Geometry: final body of the model. Coordinates: model frame, mm. A direction names the side the tool comes from. Coordinates: 2 decimals unless noted, no trailing zeros. Write each loop counter-clockwise with the first axis right and the second up, starting at its lowest first coordinate (ties: lowest second). Pieces come first, ordered by that corner, then holes. Notation, with made-up numbers: (8, 23.25) - (30, 23.25) arc R20 ccw to (30, 54.25) - close; hole circle Ø4 at (-13.5, 35). An arc over 180 degrees is marked (long way). Answer as a JSON object with one key per item and string values. Group by question number.
Item 1: Set-up query: faces 1 (the flat face through (7, 12.5, 0)), 2 (the flat face through (1, -35, 4)), 3 (the flat face through (7, 15, -29)). Return all of +Z, -Z, +X, -X, +Y, -Y with unobstructed straight access to the full face (end or side cutting, diameter ignored); none if empty.
Item 2: Section A-A on y = -25. Return loops of the section in (x, z).
Item 3: First-contact query: pin 1 Ø1.5 at (x, z) = (-5.5, -24) entering from -Y; pin 2 Ø10 at (x, z) = (1.5, -12.5) entering from -Y; pin 3 Ø6 at (x, z) = (0, 0) entering from +Y. Flat tips, straight axial feed; report the tip coordinate or a pass-through.
Item 4: Mould query, pull axis Z, two halves, no side actions, for faces 4 (the flat face through (-9.5, 1, 16.7)), 5 (the flat face through (0, -19, 30.5)), 6 (the flat face through (-7, 6, 4.5)). Classes: pulls with the +Z half, pulls with the -Z half, needs draft (parallel to the pull), parting line crosses it, or undercut.
Item 5: Section B-B on y = -39. Return loops of the section in (x, z), and give its area (3 significant figures).
Item 6: Line query: line 1 along X through (y, z) = (7, -6.5); line 2 along Y through (x, z) = (0.5, 17); line 3 along Z through (x, y) = (0, -40.25). Output: solid intervals per line, ascending. Write a range as from..to.
Item 7: Section C-C on z = 12.5. Return loops of the section in (x, y), and give its area (4 significant figures).
Autodesk Inventor part; units mm, degrees
ref_plane "YZ Plane" through (0, 0, 0) normal (1, 0, 0) x (0, 1, 0)
ref_plane "XZ Plane" through (0, 0, 0) normal (0, 1, 0) x (-1, 0, 0)
ref_plane "XY Plane" through (0, 0, 0) normal (0, 0, 1) x (1, 0, 0)
sketch "Sketch1" plane through (0, 0, 0) normal (0, 1, 0) x (-1, 0, 0)
  line L0 (6, 30.5) -> (-6, 30.5)
  line L1 (-6, 30.5) -> (-6, -30.5)
  line L2 (-6, -30.5) -> (6, -30.5)
  line L3 (6, -30.5) -> (6, 30.5)
  line L4 (8.5, 30.5) -> (-8.5, 30.5)
  line L5 (-8.5, 30.5) -> (-8.5, -30.5)
  line L6 (-8.5, -30.5) -> (8.5, -30.5)
  line L7 (8.5, -30.5) -> (8.5, 30.5)
  point P0 (0, 0)
  point P1 (-6, 30.5)
  dimension "d0" = 61
  dimension "d1" = 30.5
  dimension "d2" = 0
  dimension "d3" = 0
  dimension "d4" = 2.5
  dimension "d5" = 2.5
  dimension "d6" = 12
  dimension "d7" = 6
extrude "Extrusion1" add sketch "Sketch1" along normal blind 15.5 contours L4 L7 L6 L3 | L1 L6 L5 L4
sketch "Sketch2" plane through (0, 0, 0) normal (0, 1, 0) x (-1, 0, 0)
  line L0 (-11.5, 28) -> (11.5, 28)
  line L1 (11.5, 28) -> (11.5, -28)
  line L2 (11.5, -28) -> (-11.5, -28)
  line L3 (-11.5, -28) -> (-11.5, 28)
  line L4 (-8.5, 30.5) -> (-8.5, -30.5)
  line L5 (8.5, -30.5) -> (8.5, 30.5)
  point P0 (0, 0)
  dimension "d10" = 56
  dimension "d11" = 28
  dimension "d12" = 3
  dimension "d13" = 3
extrude "Extrusion2" add sketch "Sketch2" against normal blind 2.5
sketch "Sketch3" plane through (0, -2.5, 0) normal (0, -1, 0) x (1, 0, 0)
  line L0 (11.5, -30.5) -> (-11.5, -30.5)
  line L1 (-11.5, -30.5) -> (-11.5, 30.5)
  line L2 (-11.5, 30.5) -> (11.5, 30.5)
  line L3 (11.5, 30.5) -> (11.5, -30.5)
  line L4 (11.5, -28) -> (11.5, 28)
  line L5 (-11.5, 28) -> (-11.5, -28)
  line L6 (-11.5, -28) -> (11.5, -28)
  line L7 (11.5, 28) -> (-11.5, 28)
  point P0 (0, 0)
  point P1 (11.5, -28)
  point P2 (-11.5, -28)
  point P3 (-11.5, 28)
  point P4 (11.5, 28)
  dimension "d16" = 0
  dimension "d17" = 0
  dimension "d18" = 2.5
  dimension "d19" = 2.5
extrude "Extrusion3" add sketch "Sketch3" along normal blind 35 and the other way blind 2.5 contours L0 L1 L6 L3 | L7 L1 L2 L3
sketch "Sketch4" plane through (0, -37.5, 0) normal (0, -1, 0) x (1, 0, 0)
  line L0 (11.5, 30.5) -> (11.5, -30.5)
  line L1 (-11.5, -30.5) -> (-11.5, 30.5)
  line L2 (11.5, -30.5) -> (-11.5, -30.5)
  line L3 (-11.5, -30.5) -> (-11.5, 30.5)
  line L4 (-11.5, 30.5) -> (11.5, 30.5)
  line L5 (11.5, 30.5) -> (11.5, -30.5)
  point P0 (0, 0)
  point P1 (-11.5, -30.5)
extrude "Extrusion4" add sketch "Sketch4" along normal blind 2.5
sketch "Sketch5" plane through (0, -40, 0) normal (0, -1, 0) x (1, 0, 0)
  circle A0 centre (0, 0) radius 6
  dimension "d26" = 12
extrude "Extrusion5" add sketch "Sketch5" along normal blind 3 and the other way blind 6
sketch "Sketch6" plane through (0, -43, 0) normal (0, -1, 0) x (1, 0, 0)
  circle A0 centre (0, 0) radius 3.75
  circle A1 centre (0, 0) radius 5
  dimension "d31" = 7.5
  dimension "d32" = 10
extrude "Extrusion6" cut sketch "Sketch6" against normal blind 8
sketch "Sketch7" plane through (0, 0, 0) normal (0, 1, 0) x (1, 0, 0)
  line L0 (-11.5, -4.5) -> (12.0053, -4.5)
  line L1 (12.0053, -4.5) -> (12.0053, 4.5)
  line L2 (12.0053, 4.5) -> (-11.5, 4.5)
  line L3 (-11.5, 4.5) -> (-11.5, -4.5)
  line L4 (-11.5, 28) -> (-11.5, -28)
  point P0 (0, 0)
  point P1 (-12, 31)
  point P2 (-12, -31)
  dimension "d35" = 0
  dimension "d36" = 9
  dimension "d37" = 4.5
extrude "Extrusion7" cut sketch "Sketch7" along normal blind 12.5
chamfer "Chamfer1" distance 2 angle 45 12 edges at (-7.25, 12.5, 4.5) (-7.25, 0, 4.5) (7.25, 0, 4.5) (7.25, 12.5, -4.5) (7.25, 12.5, 4.5) (-7.25, 12.5, -4.5) (7.25, 0, -4.5) (-7.25, 0, -4.5) (8.5, 0, 17.5) (8.5, 0, -17.5) (-8.5, 0, -17.5) (-8.5, 0, 17.5)
chamfer "Chamfer2" distance 2 angle 45 4 edges at (-7.25, 15.5, 30.5) (7.25, 15.5, 30.5) (-7.25, 15.5, -30.5) (7.25, 15.5, -30.5)
fillet "Fillet1" radius 3 2 edges at (-6, -40, 0) (-6, -37.5, 0)
sketch "Sketch10" plane through (11.5, 0, 30.5) normal (1, 0, 0) x (0, 0, -1)
  line L0 (0, 0) -> (0, -40)
  line L1 (2.5, -37.5) -> (2.5, -2.5)
  line L2 (0, -40) -> (2.5, -37.5)
  line L3 (58.5, -2.5) -> (58.5, -37.5)
  line L4 (2.5, -37.5) -> (58.5, -2.5)
  line L5 (61, 0) -> (61, -40)
  line L6 (58.5, -2.5) -> (61, 0)
  line L7 (61, 0) -> (69.672, -53.3691)
  line L8 (69.672, -53.3691) -> (66.4417, -53.894)
  line L9 (66.4417, -53.894) -> (0, -40)
  line L10 (0, -40) -> (-4.0587, 20.5845)
  line L11 (-4.0587, 20.5845) -> (67.1806, 19.3093)
  arc A0 (67.1806, 19.3093) -> (69.2094, 15.0199) centre (72.5272, 19.2136) ccw
  line L12 (61, 0) -> (33, 0)
  line L13 (69.2094, 15.0199) -> (61, 0)
  point P0 (30.5, 0)
properties part number "Koszyk_v2"
Checks:
{
 "1": {"face 1": "+X, -X", "face 2": "-Y", "face 3": "-Z, +X, -X, +Y"},
 "2": {"outline": "(-11.5, -30.5) - (11.5, -30.5) - (11.5, -28) - (-11.5, -28) - close; (-11.5, 28) - (11.5, 28) - (11.5, 30.5) - (-11.5, 30.5) - close"},
 "3": {"pin 1": "y = -40", "pin 2": "y = -40.35", "pin 3": "y = 0"},
 "4": {"face 4": "needs draft", "face 5": "pulls with the +Z half", "face 6": "undercut"},
 "5": {"outline": "(-11.5, -30.5) - (11.5, -30.5) - (11.5, 30.5) - (-11.5, 30.5) - close; circle Ø7.5 at (0, 0); hole circle Ø10 at (0, 0)", "area": "1,370 mm^2"},
 "6": {"line 1": "-8.5..-6, 6..8.5", "line 2": "-40..-37.5, -2.5..0", "line 3": "-7.8..-5, -3.75..3.75, 5..7.8"},
 "7": {"outline": "(-11.5, -40) - (11.5, -40) - (11.5, -37.5) - (-11.5, -37.5) - close; (-11.5, -2.5) - (11.5, -2.5) - (11.5, 0) - (10.5, 0) - (8.5, 2) - (8.5, 15.5) - (6, 15.5) - (6, 0) - (-6, 0) - (-6, 15.5) - (-8.5, 15.5) - (-8.5, 2) - (-10.5, 0) - (-11.5, 0) - close", "area": "196.5 mm^2"}
}
